Geometry check sheet. Reference: the model listing, model coordinates, mm. Give positions to 0.01 mm unless a question says otherwise; leave off trailing zeros. Order: outer loops, then holes, each group sorted by start corner. A loop starts at its lowest first (then second) coordinate and runs counter-clockwise, first axis right, second up.
Autodesk Inventor part; units mm, degrees
ref_plane "YZ Plane" through (0, 0, 0) normal (1, 0, 0) x (0, 1, 0)
ref_plane "XZ Plane" through (0, 0, 0) normal (0, 1, 0) x (-1, 0, 0)
ref_plane "XY Plane" through (0, 0, 0) normal (0, 0, 1) x (1, 0, 0)
sketch "Sketch1" plane through (0, 0, 0) normal (0, 0, 1) x (1, 0, 0)
  line L0 (30.48, -47.625) -> (-30.48, -47.625) construction
  line L1 (-34.925, -43.18) -> (-34.925, 43.18) construction
  line L2 (-30.48, 47.625) -> (30.48, 47.625) construction
  line L3 (34.925, 43.18) -> (34.925, -43.18) construction
  line L4 (34.925, -47.625) -> (-34.925, 47.625) construction
  line L5 (-34.925, -47.625) -> (34.925, 47.625) construction
  arc A0 (-30.48, 47.625) -> (-34.925, 43.18) centre (-30.48, 43.18) ccw construction
  arc A1 (34.925, 43.18) -> (30.48, 47.625) centre (30.48, 43.18) ccw construction
  arc A2 (30.48, -47.625) -> (34.925, -43.18) centre (30.48, -43.18) ccw construction
  arc A3 (-34.925, -43.18) -> (-30.48, -47.625) centre (-30.48, -43.18) ccw construction
  circle A4 centre (-30.48, 43.18) radius 1.5
  circle A5 centre (30.48, 43.18) radius 1.5
  circle A6 centre (-30.48, -43.18) radius 1.5
  circle A7 centre (30.48, -43.18) radius 1.5
  circle A8 centre (0, -22.86) radius 6.35
  line L6 (-3.175, -7.62) -> (3.175, -7.62) construction
  line L7 (-3.175, -12.065) -> (3.175, -12.065)
  line L8 (3.175, -3.175) -> (-3.175, -3.175)
  arc A9 (-3.175, -3.175) -> (-3.175, -12.065) centre (-3.175, -7.62) ccw
  arc A10 (3.175, -12.065) -> (3.175, -3.175) centre (3.175, -7.62) ccw
  line L9 (-35.3, 57.15) -> (35.3, 57.15) construction
  line L10 (35.3, 57.15) -> (35.3, 106.85) construction
  line L11 (35.3, 106.85) -> (-35.3, 106.85) construction
  line L12 (-35.3, 106.85) -> (-35.3, 57.15) construction
  circle A11 centre (-33.25, 104.75) radius 1.25
  circle A12 centre (33.25, 104.75) radius 1.25
  circle A13 centre (33.25, 59.25) radius 1.25
  circle A14 centre (-33.25, 59.25) radius 1.25
  line L13 (-41.275, 110.025) -> (41.275, 110.025)
  line L14 (47.625, 103.675) -> (47.625, -44.45)
  line L15 (41.275, -50.8) -> (-41.275, -50.8)
  line L16 (-47.625, -44.45) -> (-47.625, 103.675)
  arc A15 (-41.275, 110.025) -> (-47.625, 103.675) centre (-41.275, 103.675) ccw
  arc A16 (47.625, 103.675) -> (41.275, 110.025) centre (41.275, 103.675) ccw
  arc A17 (41.275, -50.8) -> (47.625, -44.45) centre (41.275, -44.45) ccw
  arc A18 (-47.625, -44.45) -> (-41.275, -50.8) centre (-41.275, -44.45) ccw
  circle A19 centre (-41.275, 103.675) radius 1.5
  circle A20 centre (-41.275, -44.45) radius 1.5
  circle A21 centre (41.275, -44.45) radius 1.5
  circle A22 centre (41.275, 103.675) radius 1.5
  line L17 (-0.635, -22.225) -> (-0.635, -20.32)
  line L18 (-0.635, -20.32) -> (-3.175, -22.86)
  line L19 (-3.175, -22.86) -> (-0.635, -25.4)
  line L20 (-0.635, -25.4) -> (-0.635, -23.495)
  line L21 (-0.635, -23.495) -> (3.175, -23.495)
  line L22 (3.175, -23.495) -> (3.175, -20.32)
  line L23 (3.175, -20.32) -> (1.905, -20.32)
  line L24 (1.905, -20.32) -> (1.905, -22.225)
  line L25 (1.905, -22.225) -> (-0.635, -22.225)
  line L26 (-2.54, -8.89) -> (2.54, -8.89)
  line L27 (2.54, -8.89) -> (2.54, -7.62)
  line L28 (2.54, -7.62) -> (0, -5.08)
  line L29 (0, -5.08) -> (-2.54, -7.62)
  line L30 (-2.54, -7.62) -> (-2.54, -8.89)
  arc A23 (-19.685, -26.035) -> (-10.795, -26.035) centre (-15.24, -26.035) ccw
  line L31 (-19.685, -19.685) -> (-19.685, -26.035)
  arc A24 (-10.795, -19.685) -> (-19.685, -19.685) centre (-15.24, -19.685) ccw
  line L32 (-10.795, -26.035) -> (-10.795, -19.685)
  line L33 (-13.97, -25.4) -> (-13.97, -20.32)
  line L34 (-13.97, -20.32) -> (-15.24, -20.32)
  line L35 (-15.24, -20.32) -> (-17.78, -22.86)
  line L36 (-17.78, -22.86) -> (-15.24, -25.4)
  line L37 (-15.24, -25.4) -> (-13.97, -25.4)
  arc A25 (3.175, -42.545) -> (3.175, -33.655) centre (3.175, -38.1) ccw
  line L38 (-3.175, -42.545) -> (3.175, -42.545)
  arc A26 (-3.175, -33.655) -> (-3.175, -42.545) centre (-3.175, -38.1) ccw
  line L39 (3.175, -33.655) -> (-3.175, -33.655)
  line L40 (2.54, -36.83) -> (-2.54, -36.83)
  line L41 (-2.54, -36.83) -> (-2.54, -38.1)
  line L42 (-2.54, -38.1) -> (0, -40.64)
  line L43 (0, -40.64) -> (2.54, -38.1)
  line L44 (2.54, -38.1) -> (2.54, -36.83)
  arc A27 (19.685, -19.685) -> (10.795, -19.685) centre (15.24, -19.685) ccw
  line L45 (19.685, -26.035) -> (19.685, -19.685)
  arc A28 (10.795, -26.035) -> (19.685, -26.035) centre (15.24, -26.035) ccw
  line L46 (10.795, -19.685) -> (10.795, -26.035)
  line L47 (13.97, -20.32) -> (13.97, -25.4)
  line L48 (13.97, -25.4) -> (15.24, -25.4)
  line L49 (15.24, -25.4) -> (17.78, -22.86)
  line L50 (17.78, -22.86) -> (15.24, -20.32)
  line L51 (15.24, -20.32) -> (13.97, -20.32)
  line L52 (5.205, 21.035) -> (16.385, 21.035) construction
  line L53 (16.385, 21.035) -> (16.385, 36.115) construction
  line L54 (16.385, 36.115) -> (5.205, 36.115) construction
  line L55 (5.205, 36.115) -> (5.205, 21.035) construction
  line L56 (5.205, 21.035) -> (16.385, 36.115) construction
  line L57 (16.385, 21.035) -> (5.205, 36.115) construction
  line L58 (20.265, 22.71) -> (29.265, 22.71) construction
  line L59 (29.265, 22.71) -> (29.265, 33.61) construction
  line L60 (29.265, 33.61) -> (20.265, 33.61) construction
  line L61 (20.265, 33.61) -> (20.265, 22.71) construction
  line L62 (-7.495, 36.115) -> (-7.495, 21.035) construction
  line L63 (3.685, 36.115) -> (-7.495, 36.115) construction
  line L64 (3.685, 21.035) -> (3.685, 36.115) construction
  line L65 (-7.495, 21.035) -> (3.685, 21.035) construction
  line L66 (-20.195, 36.115) -> (-20.195, 21.035) construction
  line L67 (-9.015, 36.115) -> (-20.195, 36.115) construction
  line L68 (-9.015, 21.035) -> (-9.015, 36.115) construction
  line L69 (-20.195, 21.035) -> (-9.015, 21.035) construction
  line L70 (-32.895, 36.115) -> (-32.895, 21.035) construction
  line L71 (-21.715, 36.115) -> (-32.895, 36.115) construction
  line L72 (-21.715, 21.035) -> (-21.715, 36.115) construction
  line L73 (-32.895, 21.035) -> (-21.715, 21.035) construction
  line L74 (-33.657, 37.385) -> (17.147, 37.385)
  line L75 (17.655, 36.877) -> (17.655, 35.388)
  line L76 (18.163, 34.88) -> (30.027, 34.88)
  line L77 (30.535, 34.372) -> (30.535, 21.948)
  line L78 (30.027, 21.44) -> (18.163, 21.44)
  line L79 (17.655, 20.932) -> (17.655, 20.273)
  line L80 (17.147, 19.765) -> (-33.657, 19.765)
  line L81 (-34.165, 20.273) -> (-34.165, 36.877)
  arc A29 (-33.657, 37.385) -> (-34.165, 36.877) centre (-33.657, 36.877) ccw
  arc A30 (17.655, 36.877) -> (17.147, 37.385) centre (17.147, 36.877) ccw
  arc A31 (17.655, 35.388) -> (18.163, 34.88) centre (18.163, 35.388) ccw
  arc A32 (30.535, 34.372) -> (30.027, 34.88) centre (30.027, 34.372) ccw
  arc A33 (30.027, 21.44) -> (30.535, 21.948) centre (30.027, 21.948) ccw
  arc A34 (18.163, 21.44) -> (17.655, 20.932) centre (18.163, 20.932) ccw
  arc A35 (17.147, 19.765) -> (17.655, 20.273) centre (17.147, 20.273) ccw
  arc A36 (-34.165, 20.273) -> (-33.657, 19.765) centre (-33.657, 20.273) ccw
  line L82 (-41.1, 50.8) -> (-38.1, 50.8)
  line L83 (-38.1, 50.8) -> (-38.1, 31.75)
  line L84 (-38.1, -38.1) -> (-41.1, -38.1)
  line L85 (-41.1, -38.1) -> (-41.1, -19.05)
  line L86 (-41.1, 31.75) -> (-38.1, 31.75)
  line L87 (-41.1, -19.05) -> (-38.1, -19.05)
  line L88 (-41.1, 31.75) -> (-41.1, 50.8)
  line L89 (-41.1, -19.05) -> (-41.1, 31.75) construction
  line L90 (-38.1, -19.05) -> (-38.1, -38.1)
  line L91 (-38.1, 31.75) -> (-38.1, -19.05) construction
  circle A37 centre (-39.6, 6.35) radius 1.5
  line L92 (0, -68.4111) -> (0, 116.4523)
  line L93 (41.1, 50.8) -> (38.1, 50.8)
  line L94 (38.1, 50.8) -> (38.1, 31.75)
  line L95 (38.1, -38.1) -> (41.1, -38.1)
  line L96 (41.1, -38.1) -> (41.1, -19.05)
  line L97 (41.1, 31.75) -> (38.1, 31.75)
  line L98 (41.1, -19.05) -> (38.1, -19.05)
  line L99 (41.1, 31.75) -> (41.1, 50.8)
  line L100 (38.1, -19.05) -> (38.1, -38.1)
  circle A38 centre (39.6, 6.35) radius 1.5
  point P0 (0, 0)
  point P1 (0, 0)
  point P2 (0, -7.62)
  point P3 (0, 57.15)
  point P4 (0, 0)
  point P5 (35.3, 82)
  point P6 (0, -8.89)
  point P7 (-13.97, -22.86)
  point P8 (0, -36.83)
  point P9 (13.97, -22.86)
  point P10 (10.795, 28.575)
  point P11 (24.765, 29.21)
  point P12 (24.765, 33.61)
  point P13 (-38.1, 6.35)
  point P14 (-39.6, 50.8)
  dimension "d0" = 69.85
  dimension "d1" = 95.25
  dimension "d2" = 4.445
  dimension "d3" = 3
  dimension "d4" = 24.765
  dimension "d5" = 12.7
  dimension "d6" = 6.35
  dimension "d7" = 8.89
  dimension "d8" = 15.24
  dimension "d9" = 70.6
  dimension "d10" = 49.7
  dimension "d11" = 9.525
  dimension "d12" = 66.5
  dimension "d13" = 33.25
  dimension "d14" = 45.5
  dimension "d15" = 22.75
  dimension "d16" = 2.5
  dimension "d17" = 3.175
  dimension "d18" = 12.7
  dimension "d19" = 3.175
  dimension "d20" = 12.7
  dimension "d21" = 6.35
  dimension "d22" = 3
  dimension "d25" = 1.27
  dimension "d26" = 1.27
  dimension "d27" = 0.635
  dimension "d28" = 0.635
  dimension "d29" = 5.08
  dimension "d30" = 2.54
  dimension "d31" = 3.81
  dimension "d32" = 3.175
  dimension "d33" = 5.08
  dimension "d34" = 1.27
  dimension "d35" = 2.54
  dimension "d38" = 360
  dimension "d42" = 11.18
  dimension "d43" = 15.08
  dimension "d44" = 19.05
  dimension "d45" = 24.13
  dimension "d54" = 6.5
  dimension "d55" = 10.9
  dimension "d56" = 9
  dimension "d57" = 10.16
  dimension "d58" = 18.415
  dimension "d61" = 12.7
  dimension "d66" = 1.27
  dimension "d67" = 1.27
  dimension "d68" = 1.27
  dimension "d69" = 1.27
  dimension "d70" = 1.27
  dimension "d71" = 1.27
  dimension "d72" = 1.27
  dimension "d73" = 0.508
  dimension "d74" = 3
  dimension "d76" = 12.7
  dimension "d77" = 88.9
  dimension "d78" = 19.05
  dimension "d79" = 19.05
  dimension "d80" = 3
  dimension "d81" = 76.2
extrude "Extrusion1" add sketch "Sketch1" along normal blind 3 contours A8 L92 L21 L22 L23 L24 L25 | A8 L92 L7 A10 L8 L80 A35 L79 A34 L78 A33 L77 A32 L76 A31 L75 A30 L74 L13 A16 L14 A17 L15 L38 A25 L39 | L92 L25 L17 L18 L19 L20 L21 A8 | A8 L92 L39 A26 L38 L15 A18 L16 A15 L13 L74 A29 L81 A36 L80 L8 A9 L7 | L92 L21 L20 L19 L18 L17 L25 | L25 L24 L23 L22 L21 L92 | L92 L26 L27 L28 L8 A10 L7 | L7 A9 L8 L92 L29 L30 L26 | L92 L40 L41 L42 L38 A26 L39 | L39 A25 L38 L92 L43 L44 L40 | L92 L28 L27 L26 | L26 L30 L29 L92 | L92 L42 L41 L40 | L40 L44 L43 L92 | L92 L74 A30 L75 A31 L76 A32 L77 A33 L78 A34 L79 A35 L80 | L80 A36 L81 A29 L74 L92 | L31 A24 L32 A23 | L37 L36 L35 L34 L33 | L45 A28 L46 A27 | L51 L50 L49 L48 L47 | L82 L83 L86 L88 | L84 L85 L87 L90 | A37 | L99 L97 L94 L93 | L100 L98 L96 L95 | A38
extrude "Extrusion2" cut sketch "Sketch1" along normal blind 0.5 contours A8 L92 L21 L22 L23 L24 L25 | L92 L25 L17 L18 L19 L20 L21 A8 | L92 L26 L27 L28 L8 A10 L7 | L7 A9 L8 L92 L29 L30 L26 | L92 L40 L41 L42 L38 A26 L39 | L39 A25 L38 L92 L43 L44 L40 | L31 A24 L32 A23 | L45 A28 L46 A27
sketch "Sketch2" plane through (0, 0, 3) normal (0, 0, 1) x (1, 0, 0)
  circle A0 centre (41.275, 103.675) radius 1.5
  circle A1 centre (41.275, -44.45) radius 1.5
  circle A2 centre (-41.275, -44.45) radius 1.5
  circle A3 centre (-41.275, 103.675) radius 1.5
  circle A4 centre (30.48, -43.18) radius 1.5
  circle A5 centre (-30.48, -43.18) radius 1.5
  circle A6 centre (30.48, 43.18) radius 1.5
  circle A7 centre (-30.48, 43.18) radius 1.5
  circle A8 centre (-33.25, 59.25) radius 1.25
  circle A9 centre (33.25, 59.25) radius 1.25
  circle A10 centre (33.25, 104.75) radius 1.25
  circle A11 centre (-33.25, 104.75) radius 1.25
  line L0 (41.275, 110.025) -> (-41.275, 110.025)
  arc A12 (-41.275, 110.025) -> (-47.625, 103.675) centre (-41.275, 103.675) ccw
  line L1 (-47.625, 103.675) -> (-47.625, -44.45)
  arc A13 (-47.625, -44.45) -> (-41.275, -50.8) centre (-41.275, -44.45) ccw
  line L2 (-41.275, -50.8) -> (41.275, -50.8)
  arc A14 (41.275, -50.8) -> (47.625, -44.45) centre (41.275, -44.45) ccw
  line L3 (47.625, -44.45) -> (47.625, 103.675)
  arc A15 (47.625, 103.675) -> (41.275, 110.025) centre (41.275, 103.675) ccw
  line L4 (-41.275, 110.125) -> (41.275, 110.125)
  arc A16 (47.725, 103.675) -> (41.275, 110.125) centre (41.275, 103.675) ccw
  line L5 (47.725, 103.675) -> (47.725, -44.45)
  arc A17 (41.275, -50.9) -> (47.725, -44.45) centre (41.275, -44.45) ccw
  line L6 (41.275, -50.9) -> (-41.275, -50.9)
  arc A18 (-47.725, -44.45) -> (-41.275, -50.9) centre (-41.275, -44.45) ccw
  line L7 (-47.725, -44.45) -> (-47.725, 103.675)
  arc A19 (-41.275, 110.125) -> (-47.725, 103.675) centre (-41.275, 103.675) ccw
  point P0 (0, 0)
  dimension "d82" = 0.1
extrude "Extrusion3" add sketch "Sketch2" against normal up to surface (3 mm away) contours L4 A16 L5 A17 L6 A18 L7 A19
equation "\"d19\" = d17"
equation "\"d20\" = d18"
equation "\"d28\" = 0.5 * d26"
equation "\"d67\" = d66"
equation "\"d68\" = d66"
equation "\"d69\" = d66"
equation "\"d70\" = d66"
equation "\"d71\" = d66"
equation "\"d72\" = d66"
equation "\"d78\" = d79"
properties part number "FrontCover"
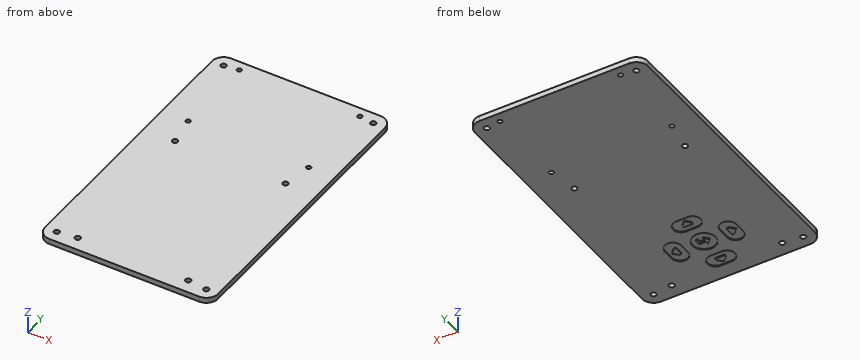
Q1. Thickness scan on L1, parallel to Y at x = -30.48, z = 2.25 (3 decimals); L2, parallel to Z at x = 0, y = -5; L3, parallel to Y at x = 40, z = 0.55 (3 decimals). Record the ranges inside material, lowest first.
Q2. Cross-section at A-A, the plane x = 30.48. Record the boundary of the cut face in (y, z) (3 decimals).
Q3. Gauge pin test, flat ends, axial feed: P1, Ø2.5, axis at x = 30.48, y = -43.18, coming from the -Z side; P2, Ø1.5, axis at x = 7, y = 81.5, coming from the -Z side. Record the tip position at first contact, or that the pin passes through.
Answers follow:
1. L1: y = -50.9 to -44.68, -41.68 to 41.68, 44.68 to 110.125
1. L2: z = 0.5 to 3
1. L3: y = -50.9 to -45.24, -43.66 to 102.885, 104.465 to 110.125
2. outline: (-50.9, 0) - (-44.68, 0) - (-44.68, 3) - (-50.9, 3) - close; (-41.68, 0) - (41.68, 0) - (41.68, 3) - (-41.68, 3) - close; (44.68, 0) - (110.125, 0) - (110.125, 3) - (44.68, 3) - close
3. P1: passes through
3. P2: stops at z = 0
